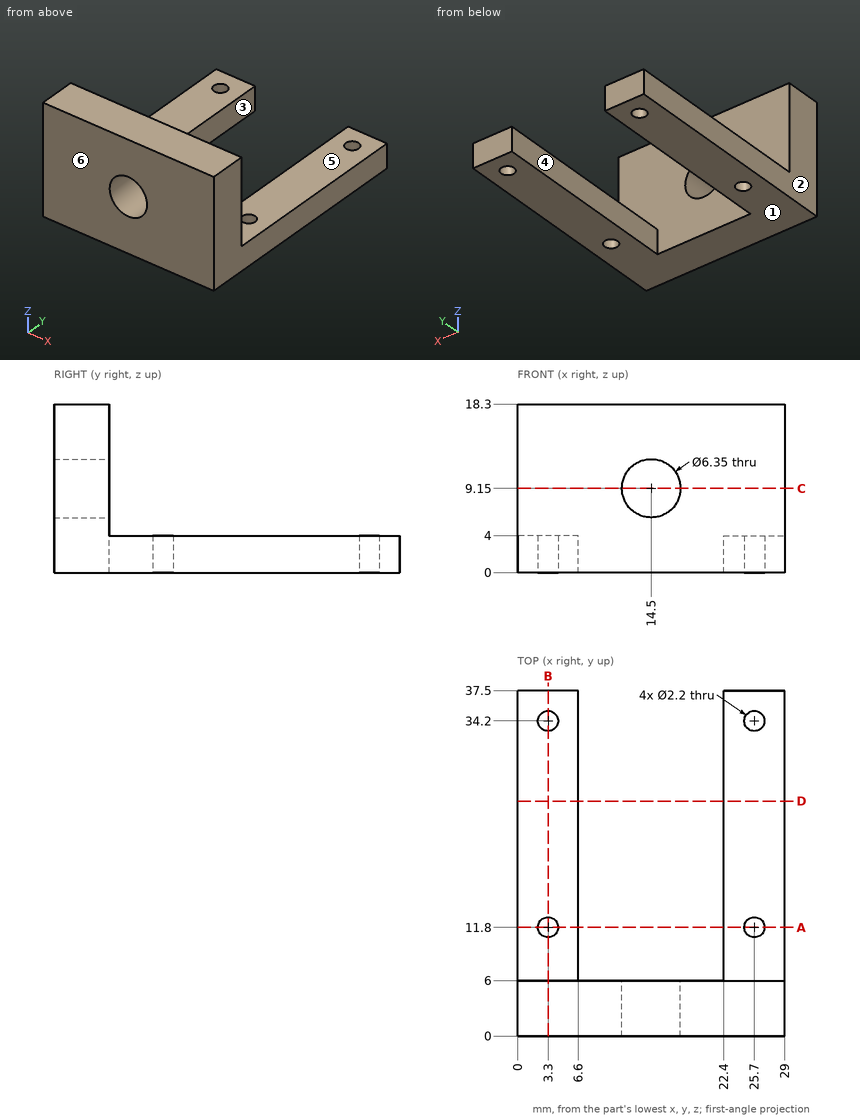
Can you work these out from the drawing? Everything is in mm from the part's minimum corner. A direction names the side the tool comes from. Give positions to 0.01 mm unless a question says otherwise; leave off trailing zeros. Write each loop counter-clockwise with the first axis right and the second up, starting at its lowest first coordinate (ties: lowest second). Pieces come first, ordered by that corner, then holes. Notation, with made-up numbers: M -35.5,-37 L -25.5,-37 A27 cw -25.5,-20 Z; hole C 11.5,34 d1. An arc over 180 degrees is marked long. Answer in a Markdown table with one row per item. Add a question column.
Item 1: We'd pull the mould along X, two halves only. Please class the marked faces 1, 2 and 3: released by +X, released by -X, zero draft, split by the parting line, or undercut.
Item 2: Imagine slicing it at D-D, the plane y = 25.5. Write out the boundary of the cut face in (x, z), plus the area to 3 significant figures.
Item 3: Imagine slicing it at C-C, the plane z = 9.15. Write out the boundary of the cut face in (x, y) (3 decimals), plus the area to 3 significant figures.
Item 4: Please list where these lines run through material, in increasing order: L1, parallel to Y at x = 25.7, z = 1.55; L2, parallel to X at y = 34.2, z = 1.6; L3, parallel to Y at x = 7.5, z = 7.5.
Item 5: Imagine slicing it at A-A, the plane y = 11.8. Write out the boundary of the cut face in (x, z), plus the area to 3 significant figures.
Item 6: On a 3-axis mill with a long thin cutter (end or side, diameter ignored), from which of +Z, -Z, +X, -X, +Y, -Y can I reach the whole of each face in a straight line? I mean the marked faces 4, 5 and 6. Say none if no direction works.
Item 7: Imagine slicing it at B-B, the plane x = 3.3. Write out the boundary of the cut face in (y, z), plus the area to 3 significant figures.
Item 8: For pin 1 Ø1 at (x, z) = (4, 11) entering from +Y; pin 2 Ø2.5 at (x, y) = (3.3, 11.8) entering from +Z, each with a flat end and sliding along its axis, tell me the tip position at first contact or that it passes through.
Evaluation:
| question | item | result |
|---|---|---|
| 1 | face 1 | zero draft |
| 1 | face 2 | released by -X |
| 1 | face 3 | undercut |
| 2 | outline | M 0,0 L 6.6,0 L 6.6,4 L 0,4 Z; M 22.4,0 L 29,0 L 29,4 L 22.4,4 Z |
| 2 | area | 52.8 mm² |
| 3 | outline | M 0,0 L 11.325,0 L 11.325,6 L 0,6 Z; M 17.675,0 L 29,0 L 29,6 L 17.675,6 Z |
| 3 | area | 136 mm² |
| 4 | L1 | y = 0 to 10.7, 12.9 to 33.1, 35.3 to 37.5 |
| 4 | L2 | x = 0 to 2.2, 4.4 to 6.6, 22.4 to 24.6, 26.8 to 29 |
| 4 | L3 | y = 0 to 6 |
| 5 | outline | M 0,0 L 2.2,0 L 2.2,4 L 0,4 Z; M 4.4,0 L 6.6,0 L 6.6,4 L 4.4,4 Z; M 22.4,0 L 24.6,0 L 24.6,4 L 22.4,4 Z; M 26.8,0 L 29,0 L 29,4 L 26.8,4 Z |
| 5 | area | 35.2 mm² |
| 6 | face 4 | +Z, -Z, +Y |
| 6 | face 5 | +Z, +X, -X, +Y |
| 6 | face 6 | +Z, -Z, +X, -X, -Y |
| 7 | outline | M 0,0 L 10.7,0 L 10.7,4 L 6,4 L 6,18.3 L 0,18.3 Z; M 12.9,0 L 33.1,0 L 33.1,4 L 12.9,4 Z; M 35.3,0 L 37.5,0 L 37.5,4 L 35.3,4 Z |
| 7 | area | 218 mm² |
| 8 | pin 1 | stops at y = 6 |
| 8 | pin 2 | stops at z = 4 |
